Read the model definition and answer for the solid it produces. Units are mm, in the model's axes. Give positions to 0.01 mm unless a question says otherwise; leave off trailing zeros. Order: outer loops, then holes, each group sorted by start corner. A loop starts at its lowest first (then second) coordinate and runs counter-clockwise, first axis right, second up. Notation, with made-up numbers: (64.5, 20) - (114.5, 20) arc R34 ccw to (114.5, 50) - close; hole circle Ø1 at (67.25, -26.75). An arc over 180 degrees is marked (long way). Write each question's results on one line, items separated by ' | '. Start each with the question number.
Q1. Find section B-B on x = -66.5. Give the vertices of the cut face in (y, z).
Q2. Find the intervals of material crossed by line 1 along Z through (x, y) = (-130, 1.5); line 2 along X through (y, z) = (2.5, -61); line 3 along X through (y, z) = (1.25, -57), in increasing order. Write a range as from..to.
Q3. Flat-ended cylindrical pins translate along their axes: P1, Ø1.5, axis at y = 1.5, z = -138.5, coming from the +X side; P2, Ø3, axis at y = 1.5, z = 41.5, coming from the -X side; P3, Ø2, axis at x = -128.5, y = 4, coming from the +Z side. Find the tip coordinate at first contact, or state that the pin passes through.
Q4. Find section A-A on y = 3.5. Give the vertices of the cut face in (x, z).
Q5. Find section C-C on z = -110.5. Give the vertices of the cut face in (x, y), and give its area (3 significant figures).
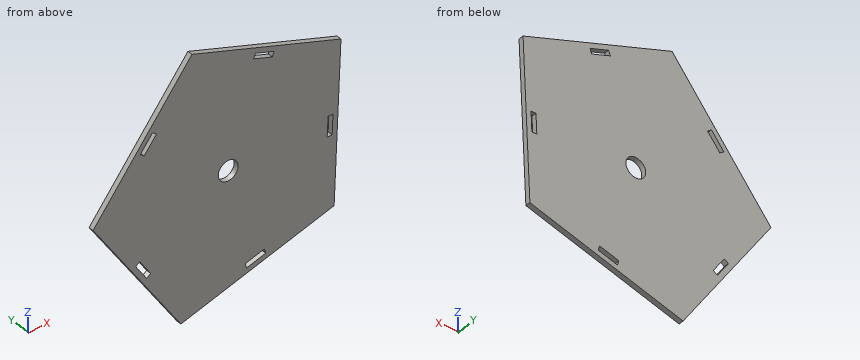
from build123d import *

# Parameters (mm, degrees)
BOSS_EXTRUDE1_DEPTH = 6.35
CUT_EXTRUDE1_DEPTH  = 7.35
SKETCH3_R           = 12.7
CUT_EXTRUDE2_DEPTH  = 7.35


with BuildPart() as part:
    # Sketch1 → Boss-Extrude1 (new body)
    with BuildSketch(Plane(origin=(0, 0, 0), x_dir=(1, 0, 0), z_dir=(0, 1, 0))):
        Polygon((-20.875255467, -32.826433561), (-29.617127229, 170.18543722), (-225.394276758, 224.605541248), (-337.649337625, 55.227144427), (-211.249631122, -103.874565796), align=None)
    extrude(amount=BOSS_EXTRUDE1_DEPTH)

    # Sketch2 → Cut-Extrude1 (cut, through all)
    with BuildSketch(Plane(origin=(0, 6.35, 0), x_dir=(1, 0, 0), z_dir=(0, 1, 0))):
        Polygon((-132.401350038, -60.892609465), (-108.604553081, -52.011592936), (-106.384298948, -57.960792175), (-130.181095905, -66.841808704), align=None)
        Polygon((-277.377537586, -10.429862968), (-261.577574273, -30.317576745), (-256.605645828, -26.367585917), (-272.405609141, -6.479872139), align=None)
        Polygon((-283.244673595, 125.822222384), (-277.951598695, 122.314251732), (-263.919716086, 143.486551334), (-269.212790987, 146.994521986), align=None)
        Polygon((-141.44240209, 194.678709813), (-116.970258399, 187.876196809), (-118.67088665, 181.758160887), (-143.143030341, 188.56067389), align=None)
        Polygon((-38.480800257, 80.821376768), (-32.136679295, 81.094560261), (-31.043945325, 55.718076413), (-37.388066287, 55.444892921), align=None)
    extrude(amount=-CUT_EXTRUDE1_DEPTH, mode=Mode.SUBTRACT)

    # Sketch3 → Cut-Extrude2 (cut, through all)
    with BuildSketch(Plane(origin=(0, 6.35, 0), x_dir=(1, 0, 0), z_dir=(0, 1, 0))):
        with Locations((-164.95712564, 62.663424707)):
            Circle(SKETCH3_R)
    extrude(amount=-CUT_EXTRUDE2_DEPTH, mode=Mode.SUBTRACT)


solid = part.part
Working result:
1) outline: (0, -180.44) - (6.35, -180.44) - (6.35, 49.85) - (0, 49.85) - close
2) line 1: -198.09..-191.5, -184.91..60, 66.77..73.55 | line 2: -333.82..-177.55, -152.37..-37.63, -31.27..-24.92 | line 3: -336.47..-176.32, -153.59..-37.46, -31.1..-24.74
3) P1: x = -28.22 | P2: x = -262 | P3: z = 73.37
4) outline: (-337.65, -55.23) - (-225.39, -224.61) - (-29.62, -170.19) - (-20.88, 32.83) - (-211.25, 103.87) - close; hole (-283.24, -125.82) - (-269.21, -146.99) - (-263.92, -143.49) - (-277.95, -122.31) - close; hole (-277.38, 10.43) - (-272.41, 6.48) - (-256.61, 26.37) - (-261.58, 30.32) - close; hole circle Ø25.4 at (-164.96, -62.66); hole (-143.14, -188.56) - (-141.44, -194.68) - (-116.97, -187.88) - (-118.67, -181.76) - close; hole (-132.4, 60.89) - (-108.6, 52.01) - (-106.38, 57.96) - (-130.18, 66.84) - close; hole (-38.48, -80.82) - (-32.14, -81.09) - (-31.04, -55.72) - (-37.39, -55.44) - close
5) outline: (-301.02, 0) - (-27.05, 0) - (-27.05, 6.35) - (-301.02, 6.35) - close | area: 1,740 mm²
